Can you work these out from the model? Positions are in its coordinate system, mm. Face numbers are marked on the shaded views. A direction names the side the tool comes from. Give positions to 0.01 mm unless a question says otherwise; leave off trailing zeros. Write each loop counter-clockwise with the first axis right and the second up, starting at its lowest first coordinate (ties: lowest second). Pieces come first, ordered by that corner, then holes. Notation, with made-up numbers: (35, -37) -> (73, -37) arc R9 cw to (73, -33) -> close; hole circle Ø10 at (55.5, 70.5). An arc over 180 degrees is marked (long way). Answer as CSV lines item,"result". Start each with the question number.
1. I'm going to push flat-ended pins straight in: P1, Ø1.6, axis at x = 23, z = -64, coming from the +Y side; P2, Ø8, axis at x = 5.5, z = -15, coming from the +Y side; P3, Ø2.5, axis at x = 42.5, z = -7.5, coming from the +Y side; P4, Ø1.2, axis at x = 6.5, z = -7.5, coming from the +Y side. Where does each tip first touch, or does it pass through?
2. On a 3-axis mill with a long thin cutter (end or side, diameter ignored), from which of +Z, -Z, +X, -X, +Y, -Y can I reach the whole of each face in a straight line? I mean the marked faces 5 and 6. Say none if no direction works.
3. If we section it at C-C on y = 3.5: Write out the boundary of the cut face in (x, z), plus the area to 3 significant figures.
4. If we section it at D-D on z = -40: Write out the boundary of the cut face in (x, y).
5. If we section it at A-A on x = 20.5: Write out the boundary of the cut face in (y, z), plus the area to 3 significant figures.
6. If we mould it in two halves opening along X, with no side actions, what happens to the marked faces 1, 2, 3 and 4? For each: pulls with the +X half, pulls with the -X half, needs draft (parallel to the pull), parting line crosses it, or undercut.
7. I need wall thicknesses on line 1 (X direction, y = 1.4, z = -7.5); line 2 (Z direction, x = 8, y = 6.25); line 3 (X direction, y = 5.5, z = -41). Which ranges of each line are inside material? Lowest first, please. Write a range as [from, to].
```python
from build123d import *

# Parameters (mm, degrees)
BOSS_EXTRUDE1_DEPTH         = 4.5
CUT_EXTRUDE1_DEPTH          = 4
SKETCH3_W                   = 13.5
SKETCH3_H                   = 6
CUT_EXTRUDE3_DEPTH          = 15
SKETCH4_R                   = 1.6
CUT_EXTRUDE4_DEPTH          = 40
SALIENTE_EXTRUIR1_START     = 4
CROQUIS1_R                  = 2
CROQUIS1_R_2                = 1.6
SALIENTE_EXTRUIR1_DEPTH     = 4
SUPERFICIE_EXTRUIR2_1_DEPTH = 2
DAR_ESPESOR1_T1             = 0.5
SALIENTE_EXTRUIR2_START     = -0.25
CROQUIS3_R                  = 1.6
SALIENTE_EXTRUIR2_DEPTH     = 0.25


with BuildPart() as part:
    # Sketch1 → Boss-Extrude1 (new body)
    with BuildSketch(Plane(origin=(0, 0, 0), x_dir=(1, 0, 0), z_dir=(0, 1, 0))):
        with BuildLine():
            Line((3.5, 0), (47, 0))
            ThreePointArc((47, 0), (49.474873734, 1.025126266), (50.5, 3.5))
            Line((50.5, 3.5), (50.5, 61.5))
            ThreePointArc((50.5, 61.5), (49.474873734, 63.974873734), (47, 65))
            Line((47, 65), (3.5, 65))
            ThreePointArc((3.5, 65), (1.025126266, 63.974873734), (0, 61.5))
            Line((0, 61.5), (0, 3.5))
            ThreePointArc((0, 3.5), (1.025126266, 1.025126266), (3.5, 0))
        make_face()
    extrude(amount=BOSS_EXTRUDE1_DEPTH)

    # Sketch2 → Cut-Extrude1 (cut)
    with BuildSketch(Plane(origin=(0, 4.5, 0), x_dir=(1, 0, 0), z_dir=(0, 1, 0))):
        with BuildLine():
            Line((5.5, 2), (45, 2))
            ThreePointArc((45, 2), (47.474873734, 3.025126266), (48.5, 5.5))
            Line((48.5, 5.5), (48.5, 59.5))
            ThreePointArc((48.5, 59.5), (47.474873734, 61.974873734), (45, 63))
            Line((45, 63), (5.5, 63))
            ThreePointArc((5.5, 63), (3.025126266, 61.974873734), (2, 59.5))
            Line((2, 59.5), (2, 5.5))
            ThreePointArc((2, 5.5), (3.025126266, 3.025126266), (5.5, 2))
        make_face()
    extrude(amount=-CUT_EXTRUDE1_DEPTH, mode=Mode.SUBTRACT)

    # Sketch3 → Cut-Extrude3 (cut)
    with BuildSketch(Plane(origin=(0, 0, -65), x_dir=(-1, 0, 0), z_dir=(0, 0, -1))):
        with Locations((-25.25, 4.5)):
            Rectangle(SKETCH3_W, SKETCH3_H)
    extrude(amount=-CUT_EXTRUDE3_DEPTH, mode=Mode.SUBTRACT)

    # Sketch4 → Cut-Extrude4 (cut)
    with BuildSketch(Plane(origin=(0, 0.5, 0), x_dir=(1, 0, 0), z_dir=(0, 1, 0))):
        with Locations(Location((6.724572176, 7.5, 0), (0, 0, 270))):
            Circle(SKETCH4_R)
        with Locations(Location((41.724572176, 7.5, 0), (0, 0, 270))):
            Circle(SKETCH4_R)
    extrude(amount=-CUT_EXTRUDE4_DEPTH, mode=Mode.SUBTRACT)

    # Croquis1 → Saliente-Extruir1 (add)
    # profile 1 of 2: a face of its own
    with BuildSketch(Plane(origin=(0, 0.5, 0), x_dir=(1, 0, 0), z_dir=(0, 1, 0)).offset(SALIENTE_EXTRUIR1_START)):
        with Locations(Location((6.724572176, 7.5, 0), (0, 0, 90))):
            Circle(CROQUIS1_R)
        with Locations(Location((6.724572176, 7.5, 0), (0, 0, 270))):
            Circle(CROQUIS1_R_2, mode=Mode.SUBTRACT)
    # profile 2 of 2: a face of its own
    with BuildSketch(Plane(origin=(0, 0.5, 0), x_dir=(1, 0, 0), z_dir=(0, 1, 0)).offset(SALIENTE_EXTRUIR1_START)):
        with Locations(Location((41.724572176, 7.5, 0), (0, 0, 90))):
            Circle(CROQUIS1_R)
        with Locations(Location((41.724572176, 7.5, 0), (0, 0, 270))):
            Circle(CROQUIS1_R_2, mode=Mode.SUBTRACT)
    extrude(amount=-SALIENTE_EXTRUIR1_DEPTH)

    # Superficie-Extruir2: a surface, the sketch's curves swept straight by 2 mm
    with BuildLine(Plane(origin=(0, 4.5, 0), x_dir=(1, 0, 0), z_dir=(0, 1, 0)), mode=Mode.PRIVATE) as superficie_extruir2_1_path:
        Line((18.5, 63), (18.5, 65))
        Line((18.5, 65), (3.5, 65))
        ThreePointArc((3.5, 65), (1.025126266, 63.974873734), (0, 61.5))
        Line((0, 61.5), (0, 3.5))
        ThreePointArc((0, 3.5), (1.025126266, 1.025126266), (3.5, 0))
        Line((3.5, 0), (47, 0))
        ThreePointArc((47, 0), (49.474873734, 1.025126266), (50.5, 3.5))
        Line((50.5, 3.5), (50.5, 61.5))
        ThreePointArc((50.5, 61.5), (49.474873734, 63.974873734), (47, 65))
        Line((47, 65), (32, 65))
        Line((32, 65), (32, 63))
        Line((32, 63), (45, 63))
        ThreePointArc((45, 63), (47.474873734, 61.974873734), (48.5, 59.5))
        Line((48.5, 59.5), (48.5, 5.5))
        ThreePointArc((48.5, 5.5), (47.474873734, 3.025126266), (45, 2))
        Line((45, 2), (5.5, 2))
        ThreePointArc((5.5, 2), (3.025126266, 3.025126266), (2, 5.5))
        Line((2, 5.5), (2, 59.5))
        ThreePointArc((2, 59.5), (3.025126266, 61.974873734), (5.5, 63))
        Line((5.5, 63), (18.5, 63))
    superficie_extruir2_1 = Shell.extrude(superficie_extruir2_1_path.wire(), (0 * SUPERFICIE_EXTRUIR2_1_DEPTH, 1 * SUPERFICIE_EXTRUIR2_1_DEPTH, 0 * SUPERFICIE_EXTRUIR2_1_DEPTH))
    add(Solid.thicken(superficie_extruir2_1, DAR_ESPESOR1_T1))

    # Croquis3 → Saliente-Extruir2 (add)
    with BuildSketch(Plane.XZ.offset(SALIENTE_EXTRUIR2_START)):
        with Locations(Location((6.724572176, -7.5, 0), (0, 0, 90))):
            Circle(CROQUIS3_R)
        with Locations(Location((41.724572176, -7.5, 0), (0, 0, 90))):
            Circle(CROQUIS3_R)
    extrude(amount=SALIENTE_EXTRUIR2_DEPTH)


solid = part.part
```
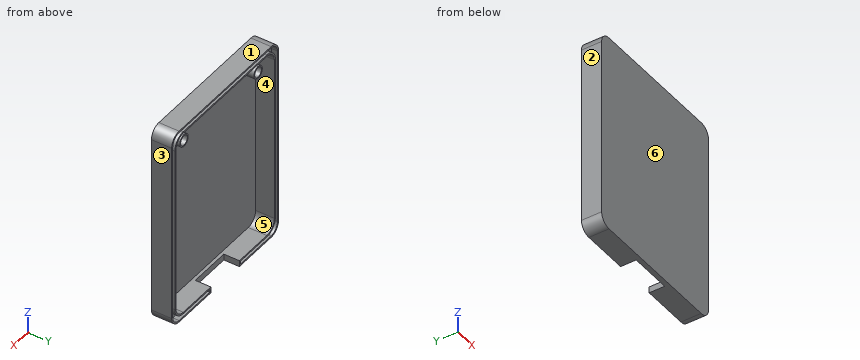
Computed values:
1,P1,"stops at y = 1.5"
1,P2,"stops at y = 6.5"
1,P3,"stops at y = 4.5"
1,P4,"stops at y = 0.25"
2,face 5,"+Y"
2,face 6,"+Z, -Z, +X, -X, -Y"
3,outline,"(0, -61.5) arc R3.5 ccw to (3.5, -65) -> (18.5, -65) -> (18.5, -63) -> (5.5, -63) arc R3.5 cw to (2, -59.5) -> (2, -5.5) arc R3.5 cw to (5.5, -2) -> (45, -2) arc R3.5 cw to (48.5, -5.5) -> (48.5, -59.5) arc R3.5 cw to (45, -63) -> (32, -63) -> (32, -65) -> (47, -65) arc R3.5 ccw to (50.5, -61.5) -> (50.5, -3.5) arc R3.5 ccw to (47, 0) -> (3.5, 0) arc R3.5 ccw to (0, -3.5) -> close; circle Ø4 at (6.72, -7.5); circle Ø4 at (41.72, -7.5); hole circle Ø3.2 at (6.72, -7.5); hole circle Ø3.2 at (41.72, -7.5)"
3,area,"428 mm2"
4,outline,"(0, 0) -> (50.5, 0) -> (50.5, 6.5) -> (50, 6.5) -> (50, 4.5) -> (49, 4.5) -> (49, 6.5) -> (48.5, 6.5) -> (48.5, 0.5) -> (2, 0.5) -> (2, 6.5) -> (1.5, 6.5) -> (1.5, 4.5) -> (0.5, 4.5) -> (0.5, 6.5) -> (0, 6.5) -> close"
5,outline,"(0, -65) -> (1.5, -65) -> (1.5, -63) -> (0.5, -63) -> (0.5, -2) -> (6.5, -2) -> (6.5, -1.5) -> (4.5, -1.5) -> (4.5, -0.5) -> (6.5, -0.5) -> (6.5, 0) -> (0, 0) -> close"
5,area,"44.5 mm2"
6,face 1,"needs draft"
6,face 2,"pulls with the -X half"
6,face 3,"pulls with the +X half"
6,face 4,"undercut"
7,line 1,"x = [0, 2], [4.72, 5.12], [8.32, 8.72], [39.72, 40.12], [43.32, 43.72], [48.5, 50.5]"
7,line 2,"z = [-65, -64.5], [-63.5, -63], [-2, -1.5], [-0.5, 0]"
7,line 3,"x = [0, 0.5], [1.5, 2], [48.5, 49], [50, 50.5]"
